from build123d import *

# Parameters (mm, degrees)
EXTRUDE_1_DEPTH     = 3
SKETCH_2_W          = 5
SKETCH_2_H          = 8
CUT_EXTRUDE_1_DEPTH = 3
SKETCH_3_R          = 1.5
CUT_EXTRUDE_2_DEPTH = 3
SKETCH_4_R          = 3
CUT_EXTRUDE_3_DEPTH = 1.6
CUT_EXTRUDE_4_REACH = 5
SKETCH_5_R          = 1.005


with BuildPart() as part:
    # 草图1 → 凸台-拉伸1 (new body)
    with BuildSketch(Plane.XY):
        Polygon((16, 0), (-16, 0), (-16, 8), (-13, 8), (-13, 16), (-16, 16), (-16, 24), (-13, 24), (-13, 32), (-16, 32), (-16, 40), (-13, 40), (-13, 48), (-16, 48), (-16, 56), (-13, 56), (-13, 64), (13, 64), (13, 56), (16, 56), (16, 48), (13, 48), (13, 40), (16, 40), (16, 32), (13, 32), (13, 24), (16, 24), (16, 16), (13, 16), (13, 8), (16, 8), align=None)
    extrude(amount=EXTRUDE_1_DEPTH)

    # 草图2 → 切除-拉伸1 (cut)
    with BuildSketch(Plane.XY.offset(3)):
        with Locations((-4, 28)):
            Rectangle(SKETCH_2_W, SKETCH_2_H)
        with Locations((-4, 12)):
            Rectangle(SKETCH_2_W, SKETCH_2_H)
        with Locations((4, 28)):
            Rectangle(SKETCH_2_W, SKETCH_2_H)
        with Locations((-4, 44)):
            Rectangle(SKETCH_2_W, SKETCH_2_H)
        with Locations((4, 44)):
            Rectangle(SKETCH_2_W, SKETCH_2_H)
        with Locations((4, 12)):
            Rectangle(SKETCH_2_W, SKETCH_2_H)
        with Locations((4, 60)):
            Rectangle(SKETCH_2_W, SKETCH_2_H)
        with Locations((-4, 60)):
            Rectangle(SKETCH_2_W, SKETCH_2_H)
    extrude(amount=-CUT_EXTRUDE_1_DEPTH, mode=Mode.SUBTRACT)

    # 草图3 → 切除-拉伸2 (cut)
    with BuildSketch(Plane.XY.offset(3)):
        with Locations((-11.4, 4)):
            Circle(SKETCH_3_R)
        with Locations((11.4, 4)):
            Circle(SKETCH_3_R)
        with Locations((-11.4, 20)):
            Circle(SKETCH_3_R)
        with Locations((11.4, 20)):
            Circle(SKETCH_3_R)
        with Locations((-11.4, 36)):
            Circle(SKETCH_3_R)
        with Locations((11.4, 36)):
            Circle(SKETCH_3_R)
        with Locations((-11.4, 52)):
            Circle(SKETCH_3_R)
        with Locations((11.4, 52)):
            Circle(SKETCH_3_R)
    extrude(amount=-CUT_EXTRUDE_2_DEPTH, mode=Mode.SUBTRACT)

    # 草图4 → 切除-拉伸3 (cut)
    with BuildSketch(Plane.XY.offset(3)):
        with Locations((-11.4, 4)):
            Circle(SKETCH_4_R)
        with Locations((11.4, 4)):
            Circle(SKETCH_4_R)
        with Locations((-11.4, 20)):
            Circle(SKETCH_4_R)
        with Locations((11.4, 20)):
            Circle(SKETCH_4_R)
        with Locations((-11.4, 36)):
            Circle(SKETCH_4_R)
        with Locations((11.4, 36)):
            Circle(SKETCH_4_R)
        with Locations((-11.4, 52)):
            Circle(SKETCH_4_R)
        with Locations((11.4, 52)):
            Circle(SKETCH_4_R)
    extrude(amount=-CUT_EXTRUDE_3_DEPTH, mode=Mode.SUBTRACT)

    # 草图5 → 切除-拉伸4 (cut, up to next)
    with BuildSketch(Plane.XY.offset(3), mode=Mode.PRIVATE) as cut_extrude_4_sk1:
        with Locations((-13, 57.005)):
            Circle(SKETCH_5_R)
    cut_extrude_4_tool1 = extrude(cut_extrude_4_sk1.sketch, amount=-CUT_EXTRUDE_4_REACH, mode=Mode.PRIVATE) & part.part
    add(cut_extrude_4_tool1.solids().sort_by_distance((-13, 57.005, 3))[0], mode=Mode.SUBTRACT)
    # 草图5 → 切除-拉伸4 (cut, up to next)
    with BuildSketch(Plane.XY.offset(3), mode=Mode.PRIVATE) as cut_extrude_4_sk2:
        with Locations((-13, 46.995)):
            Circle(SKETCH_5_R)
    cut_extrude_4_tool2 = extrude(cut_extrude_4_sk2.sketch, amount=-CUT_EXTRUDE_4_REACH, mode=Mode.PRIVATE) & part.part
    add(cut_extrude_4_tool2.solids().sort_by_distance((-13, 46.995, 3))[0], mode=Mode.SUBTRACT)
    # 草图5 → 切除-拉伸4 (cut, up to next)
    with BuildSketch(Plane.XY.offset(3), mode=Mode.PRIVATE) as cut_extrude_4_sk3:
        with Locations((-13, 41.005)):
            Circle(SKETCH_5_R)
    cut_extrude_4_tool3 = extrude(cut_extrude_4_sk3.sketch, amount=-CUT_EXTRUDE_4_REACH, mode=Mode.PRIVATE) & part.part
    add(cut_extrude_4_tool3.solids().sort_by_distance((-13, 41.005, 3))[0], mode=Mode.SUBTRACT)
    # 草图5 → 切除-拉伸4 (cut, up to next)
    with BuildSketch(Plane.XY.offset(3), mode=Mode.PRIVATE) as cut_extrude_4_sk4:
        with Locations((-13, 30.995)):
            Circle(SKETCH_5_R)
    cut_extrude_4_tool4 = extrude(cut_extrude_4_sk4.sketch, amount=-CUT_EXTRUDE_4_REACH, mode=Mode.PRIVATE) & part.part
    add(cut_extrude_4_tool4.solids().sort_by_distance((-13, 30.995, 3))[0], mode=Mode.SUBTRACT)
    # 草图5 → 切除-拉伸4 (cut, up to next)
    with BuildSketch(Plane.XY.offset(3), mode=Mode.PRIVATE) as cut_extrude_4_sk5:
        with Locations((-13, 25.005)):
            Circle(SKETCH_5_R)
    cut_extrude_4_tool5 = extrude(cut_extrude_4_sk5.sketch, amount=-CUT_EXTRUDE_4_REACH, mode=Mode.PRIVATE) & part.part
    add(cut_extrude_4_tool5.solids().sort_by_distance((-13, 25.005, 3))[0], mode=Mode.SUBTRACT)
    # 草图5 → 切除-拉伸4 (cut, up to next)
    with BuildSketch(Plane.XY.offset(3), mode=Mode.PRIVATE) as cut_extrude_4_sk6:
        with Locations((-13, 14.995)):
            Circle(SKETCH_5_R)
    cut_extrude_4_tool6 = extrude(cut_extrude_4_sk6.sketch, amount=-CUT_EXTRUDE_4_REACH, mode=Mode.PRIVATE) & part.part
    add(cut_extrude_4_tool6.solids().sort_by_distance((-13, 14.995, 3))[0], mode=Mode.SUBTRACT)
    # 草图5 → 切除-拉伸4 (cut, up to next)
    with BuildSketch(Plane.XY.offset(3), mode=Mode.PRIVATE) as cut_extrude_4_sk7:
        with Locations((-13, 9.005)):
            Circle(SKETCH_5_R)
    cut_extrude_4_tool7 = extrude(cut_extrude_4_sk7.sketch, amount=-CUT_EXTRUDE_4_REACH, mode=Mode.PRIVATE) & part.part
    add(cut_extrude_4_tool7.solids().sort_by_distance((-13, 9.005, 3))[0], mode=Mode.SUBTRACT)
    # 草图5 → 切除-拉伸4 (cut, up to next)
    with BuildSketch(Plane.XY.offset(3), mode=Mode.PRIVATE) as cut_extrude_4_sk8:
        with Locations((13, 9.005)):
            Circle(SKETCH_5_R)
    cut_extrude_4_tool8 = extrude(cut_extrude_4_sk8.sketch, amount=-CUT_EXTRUDE_4_REACH, mode=Mode.PRIVATE) & part.part
    add(cut_extrude_4_tool8.solids().sort_by_distance((13, 9.005, 3))[0], mode=Mode.SUBTRACT)
    # 草图5 → 切除-拉伸4 (cut, up to next)
    with BuildSketch(Plane.XY.offset(3), mode=Mode.PRIVATE) as cut_extrude_4_sk9:
        with Locations((13, 14.995)):
            Circle(SKETCH_5_R)
    cut_extrude_4_tool9 = extrude(cut_extrude_4_sk9.sketch, amount=-CUT_EXTRUDE_4_REACH, mode=Mode.PRIVATE) & part.part
    add(cut_extrude_4_tool9.solids().sort_by_distance((13, 14.995, 3))[0], mode=Mode.SUBTRACT)
    # 草图5 → 切除-拉伸4 (cut, up to next)
    with BuildSketch(Plane.XY.offset(3), mode=Mode.PRIVATE) as cut_extrude_4_sk10:
        with Locations((13, 25.005)):
            Circle(SKETCH_5_R)
    cut_extrude_4_tool10 = extrude(cut_extrude_4_sk10.sketch, amount=-CUT_EXTRUDE_4_REACH, mode=Mode.PRIVATE) & part.part
    add(cut_extrude_4_tool10.solids().sort_by_distance((13, 25.005, 3))[0], mode=Mode.SUBTRACT)
    # 草图5 → 切除-拉伸4 (cut, up to next)
    with BuildSketch(Plane.XY.offset(3), mode=Mode.PRIVATE) as cut_extrude_4_sk11:
        with Locations((13, 30.995)):
            Circle(SKETCH_5_R)
    cut_extrude_4_tool11 = extrude(cut_extrude_4_sk11.sketch, amount=-CUT_EXTRUDE_4_REACH, mode=Mode.PRIVATE) & part.part
    add(cut_extrude_4_tool11.solids().sort_by_distance((13, 30.995, 3))[0], mode=Mode.SUBTRACT)
    # 草图5 → 切除-拉伸4 (cut, up to next)
    with BuildSketch(Plane.XY.offset(3), mode=Mode.PRIVATE) as cut_extrude_4_sk12:
        with Locations((13, 41.005)):
            Circle(SKETCH_5_R)
    cut_extrude_4_tool12 = extrude(cut_extrude_4_sk12.sketch, amount=-CUT_EXTRUDE_4_REACH, mode=Mode.PRIVATE) & part.part
    add(cut_extrude_4_tool12.solids().sort_by_distance((13, 41.005, 3))[0], mode=Mode.SUBTRACT)
    # 草图5 → 切除-拉伸4 (cut, up to next)
    with BuildSketch(Plane.XY.offset(3), mode=Mode.PRIVATE) as cut_extrude_4_sk13:
        with Locations((13, 46.995)):
            Circle(SKETCH_5_R)
    cut_extrude_4_tool13 = extrude(cut_extrude_4_sk13.sketch, amount=-CUT_EXTRUDE_4_REACH, mode=Mode.PRIVATE) & part.part
    add(cut_extrude_4_tool13.solids().sort_by_distance((13, 46.995, 3))[0], mode=Mode.SUBTRACT)
    # 草图5 → 切除-拉伸4 (cut, up to next)
    with BuildSketch(Plane.XY.offset(3), mode=Mode.PRIVATE) as cut_extrude_4_sk14:
        with Locations((13, 57.005)):
            Circle(SKETCH_5_R)
    cut_extrude_4_tool14 = extrude(cut_extrude_4_sk14.sketch, amount=-CUT_EXTRUDE_4_REACH, mode=Mode.PRIVATE) & part.part
    add(cut_extrude_4_tool14.solids().sort_by_distance((13, 57.005, 3))[0], mode=Mode.SUBTRACT)


solid = part.part
Source: CAD feature listing. Evaluate the final solid. Frame: model axes, mm. A direction names the side the tool comes from. Round coordinates to 2 decimals unless told otherwise and drop trailing zeros. Order: outer loops, then holes, each group sorted by start corner. A loop starts at its lowest first (then second) coordinate and runs counter-clockwise, first axis right, second up. Notation, with made-up numbers: (-3.75, 11.25) - (0.25, 11.25) arc R11 cw to (0.25, 23.25) - close; hole circle Ø10 at (-32, -10.5). An arc over 180 degrees is marked (long way). Use a Markdown table: item, result. Add a question column.
1. Mould query, pull axis X, two halves, no side actions, for faces 1 (the flat face through (10, 35, 1.4)), 2 (the flat face through (-6.5, 12, 2)), 3 (the flat face through (-13, 61, 1)), 4 (the flat face through (14, 56, 1)). Classes: +X half, -X half, draft (parallel to the pull), parting line (faces both ways), or undercut.
2. Section query B-B (x = -5). Return the cut outline in (y, z), then the cut area to 3 significant figures.
3. Section query C-C (x = 11.4). Give the number of separate pieces and of enclosed holes in the cut face, then the cut area to 3 significant figures.
4. First-contact query: pin 1 (0.9 mm diameter, centred on x = 5, z = 1, fed in from +Y); pin 2 (1.5 mm diameter, centred on y = 28, z = 1, fed in from -X); pin 3 (5 mm diameter, centred on x = 11.4, y = 36, fed in from +Z). Flat tips, straight axial feed; report the tip coordinate or a pass-through.
5. Section query A-A (y = 4). Return the cut outline in (x, z).
6. Set-up query: faces 5 (the flat face through (15, 16, 1)), 6 (the flat face through (-13, 12, 1)), 7 (the flat face through (10, 3, 1.4)), 8 (the flat face through (-4, 8, 2)). Return all of +Z, -Z, +X, -X, +Y, -Y with unobstructed straight access to the full face (end or side cutting, diameter ignored); none if empty.
7. Line query: probe 1 along Y at (x, z) = (5, 2.65); probe 2 along X at (y, z) = (11.5, 2.2); probe 3 along Y at (x, z) = (-11.4, 1.75). Output: solid intervals per line, ascending.
Derived:
| question | item | result |
|---|---|---|
| 1 | face 1 | undercut |
| 1 | face 2 | undercut |
| 1 | face 3 | -X half |
| 1 | face 4 | draft |
| 2 | outline | (0, 0) - (8, 0) - (8, 3) - (0, 3) - close; (16, 0) - (24, 0) - (24, 3) - (16, 3) - close; (32, 0) - (40, 0) - (40, 3) - (32, 3) - close; (48, 0) - (56, 0) - (56, 3) - (48, 3) - close |
| 2 | area | 96.0 mm2 |
| 3 | separate pieces | 5 |
| 3 | enclosed holes | 0 |
| 3 | area | 137 mm2 |
| 4 | pin 1 | y = 56 |
| 4 | pin 2 | x = -13 |
| 4 | pin 3 | z = 1.4 |
| 5 | outline | (-16, 0) - (-12.9, 0) - (-12.9, 1.4) - (-14.4, 1.4) - (-14.4, 3) - (-16, 3) - close; (-9.9, 0) - (9.9, 0) - (9.9, 1.4) - (8.4, 1.4) - (8.4, 3) - (-8.4, 3) - (-8.4, 1.4) - (-9.9, 1.4) - close; (12.9, 0) - (16, 0) - (16, 3) - (14.4, 3) - (14.4, 1.4) - (12.9, 1.4) - close |
| 6 | face 5 | +Z, -Z, +X |
| 6 | face 6 | +Z, -Z, -X |
| 6 | face 7 | +Z |
| 6 | face 8 | +Z, -Z |
| 7 | probe 1 | 0 to 8, 16 to 24, 32 to 40, 48 to 56 |
| 7 | probe 2 | -13 to -6.5, -1.5 to 1.5, 6.5 to 13 |
| 7 | probe 3 | 0 to 1, 7 to 17, 23 to 33, 39 to 49, 55 to 64 |
